```python
from build123d import *

# Parameters (mm, degrees)
SKETCH1_W           = 160
SKETCH1_H           = 100
BOSS_EXTRUDE2_DEPTH = 50
CUT_EXTRUDE2_DEPTH  = 50
CUT_EXTRUDE3_DEPTH  = 50
CUT_EXTRUDE4_DEPTH  = 20
CUT_EXTRUDE5_DEPTH  = 20
SKETCH8_W           = 40
SKETCH8_H           = 10
CUT_EXTRUDE6_DEPTH  = 125
SKETCH9_R           = 35
BOSS_EXTRUDE3_DEPTH = 10
SKETCH10_R          = 15
CUT_EXTRUDE8_DEPTH  = 123
SKETCH11_R          = 35
BOSS_EXTRUDE4_DEPTH = 30
SKETCH12_R          = 15
CUT_EXTRUDE9_DEPTH  = 30
SKETCH13_R          = 20
CUT_EXTRUDE10_DEPTH = 30
CUT_EXTRUDE11_DEPTH = 20
SKETCH15_R          = 20
SKETCH15_R_2        = 15
CUT_EXTRUDE12_DEPTH = 10


with BuildPart() as part:
    # Sketch1 → Boss-Extrude2 (new body)
    with BuildSketch(Plane.XY):
        with Locations((80, 50)):
            Rectangle(SKETCH1_W, SKETCH1_H)
    extrude(amount=BOSS_EXTRUDE2_DEPTH)

    # Sketch4 → Cut-Extrude2 (cut)
    with BuildSketch(Plane.XY.offset(50)):
        Polygon((0, 80), (20, 100), (0, 100), align=None)
        Polygon((0, 20), (20, 0), (0, 0), align=None)
        Polygon((140, 100), (160, 80), (160, 100), align=None)
        Polygon((160, 20), (140, 0), (160, 0), align=None)
    extrude(amount=-CUT_EXTRUDE2_DEPTH, mode=Mode.SUBTRACT)

    # Sketch5 → Cut-Extrude3 (cut)
    with BuildSketch(Plane.XY.offset(50)):
        Polygon((10, 70), (0, 70), (0, 30), (10, 30), (10, 40), (30, 40), (30, 60), (10, 60), align=None)
        Polygon((160, 30), (160, 70), (150, 70), (150, 60), (130, 60), (130, 40), (150, 40), (150, 30), align=None)
    extrude(amount=-CUT_EXTRUDE3_DEPTH, mode=Mode.SUBTRACT)

    # Sketch6 → Cut-Extrude4 (cut)
    with BuildSketch(Plane.XY.offset(50)):
        Polygon((10, 70), (40, 70), (40, 30), (10, 30), (10, 40), (30, 40), (30, 60), (10, 60), align=None)
    extrude(amount=-CUT_EXTRUDE4_DEPTH, mode=Mode.SUBTRACT)

    # Sketch7 → Cut-Extrude5 (cut)
    with BuildSketch(Plane.XY.offset(50)):
        Polygon((150, 70), (120, 70), (120, 30), (150, 30), (150, 40), (130, 40), (130, 60), (150, 60), align=None)
    extrude(amount=-CUT_EXTRUDE5_DEPTH, mode=Mode.SUBTRACT)

    # Sketch8 → Cut-Extrude6 (cut)
    with BuildSketch(Plane.XY.offset(50)):
        with Locations((80, 95)):
            Rectangle(SKETCH8_W, SKETCH8_H)
        with Locations((80, 5)):
            Rectangle(SKETCH8_W, SKETCH8_H)
    extrude(amount=-CUT_EXTRUDE6_DEPTH, mode=Mode.SUBTRACT)

    # Sketch9 → Boss-Extrude3 (add)
    with BuildSketch(Plane(origin=(0, 0, 0), x_dir=(-1, 0, 0), z_dir=(0, 0, -1))):
        with Locations((-80, 50)):
            Circle(SKETCH9_R)
    extrude(amount=BOSS_EXTRUDE3_DEPTH)

    # Sketch10 → Cut-Extrude8 (cut)
    with BuildSketch(Plane(origin=(0, 0, -10), x_dir=(-1, 0, 0), z_dir=(0, 0, -1))):
        with Locations((-80, 50)):
            Circle(SKETCH10_R)
    extrude(amount=-CUT_EXTRUDE8_DEPTH, mode=Mode.SUBTRACT)

    # Sketch11 → Boss-Extrude4 (add)
    with BuildSketch(Plane.XY.offset(50)):
        with Locations((80, 50)):
            Circle(SKETCH11_R)
    extrude(amount=BOSS_EXTRUDE4_DEPTH)

    # Sketch12 → Cut-Extrude9 (cut)
    with BuildSketch(Plane(origin=(0, 0, 50), x_dir=(-1, 0, 0), z_dir=(0, 0, -1))):
        with Locations((-80, 50)):
            Circle(SKETCH12_R)
    extrude(amount=-CUT_EXTRUDE9_DEPTH, mode=Mode.SUBTRACT)

    # Sketch13 → Cut-Extrude10 (cut)
    with BuildSketch(Plane.XY.offset(80)):
        with Locations((80, 50)):
            Circle(SKETCH13_R)
    extrude(amount=-CUT_EXTRUDE10_DEPTH, mode=Mode.SUBTRACT)

    # Sketch14 → Cut-Extrude11 (cut)
    with BuildSketch(Plane.XY.offset(80)):
        with BuildLine():
            ThreePointArc((66.771243445, 35), (60, 50), (66.771243445, 65))
            Line((66.771243445, 65), (48.377223398, 65))
            ThreePointArc((48.377223398, 65), (45, 50), (48.377223398, 35))
            Line((48.377223398, 35), (66.771243445, 35))
        make_face()
        with BuildLine():
            Line((111.622776602, 65), (93.228756555, 65))
            ThreePointArc((93.228756555, 65), (98.228756555, 58.228756555), (100, 50))
            ThreePointArc((100, 50), (98.228756555, 41.771243445), (93.228756555, 35))
            Line((93.228756555, 35), (111.622776602, 35))
            ThreePointArc((111.622776602, 35), (114.145257219, 42.312255892), (115, 50))
            ThreePointArc((115, 50), (114.145257219, 57.687744108), (111.622776602, 65))
        make_face()
    extrude(amount=-CUT_EXTRUDE11_DEPTH, mode=Mode.SUBTRACT)

    # Sketch15 → Cut-Extrude12 (cut)
    with BuildSketch(Plane.XY.offset(50)):
        with Locations((80, 50)):
            Circle(SKETCH15_R)
        with Locations((80, 50)):
            Circle(SKETCH15_R_2, mode=Mode.SUBTRACT)
    extrude(amount=-CUT_EXTRUDE12_DEPTH, mode=Mode.SUBTRACT)


solid = part.part
```
For this review, take the finished solid that the model builds, in its own axes (mm). A direction names the side the tool comes from. Coordinates: 2 decimals unless noted, no trailing zeros. Loops run counter-clockwise (first coordinate to the right, second up) from the corner with the lowest first, then second, coordinate; pieces in that order, holes last.
1. Add section B-B, the plane x = 16.5. Give the boundary of the cut face in (y, z), then the cut area to 3 significant figures.
2. Add section D-D, the plane z = 35.5. Give the boundary of the cut face in (x, y), then the cut area to 3 significant figures.
3. Add section A-A, the plane z = 73.5. Give the boundary of the cut face in (x, y), then the cut area to 3 significant figures.
4. Insertion check: P1, Ø3, axis at y = 4, z = 19, coming from the +X side; P2, Ø3, axis at y = 37, z = 12.5, coming from the +X side; P3, Ø22, axis at x = 21.5, z = 17.5, coming from the -Y side; P4, Ø1.5, axis at y = 69.5, z = 59.5, coming from the +X side. Each pin has a flat end and moves straight along its axis. Give the tip position at first contact, or say it passes through.
5. For faces 1 (the flat face through (128, 50, 30)), 2 (the flat face through (100, 5, 25)), 3 (the flat face through (103, 65, 70)), 4 (the flat face through (30, 50, 15)), 5 (the flat face through (150, 35, 15)), list the 3-axis set-ups (+Z, -Z, +X, -X, +Y, -Y) from which the entire face can be reached by the end or side of a thin tool; tool diameter is ignored.
6. For line 1 (X direction, y = 50, z = 56); line 2 (Y direction, x = 80, z = 61.5); line 3 (Y direction, x = 80, z = 11), list the stretches that pass through material, from the lowest coordinate up.
7. Add section C-C, the plane y = 50. Give the boundary of the cut face in (x, z).
8. Mouldability with a two-part tool opening along Y and no side actions: class faces 6 (the flat face through (145, 70, 36)), 7 (the cylindrical face through (61.18, 79.51, -4.93)), 8 (the flat face through (160, 75, 25)), 9 (the cylindrical face through (71.94, 62.65, 14.65)) as +Y half, -Y half, draft (parallel to the pull), parting line (faces both ways), or undercut.
Result:
1. outline: (3.5, 0) - (40, 0) - (40, 30) - (30, 30) - (30, 50) - (3.5, 50) - close; (60, 0) - (96.5, 0) - (96.5, 50) - (70, 50) - (70, 30) - (60, 30) - close
1. area: 3,250 mm2
2. outline: (0, 20) - (20, 0) - (60, 0) - (60, 10) - (100, 10) - (100, 0) - (140, 0) - (160, 20) - (160, 30) - (120, 30) - (120, 70) - (160, 70) - (160, 80) - (140, 100) - (100, 100) - (100, 90) - (60, 90) - (60, 100) - (20, 100) - (0, 80) - (0, 70) - (40, 70) - (40, 30) - (0, 30) - close; hole circle Ø30 at (80, 50)
2. area: 10,500 mm2
3. outline: (48.38, 35) arc R35 ccw to (111.62, 35) - (93.23, 35) arc R20 cw to (66.77, 35) - close; (48.38, 65) - (66.77, 65) arc R20 cw to (93.23, 65) - (111.62, 65) arc R35 ccw to start
3. area: 1,630 mm2
4. P1: stops at x = 145.5
4. P2: stops at x = 150
4. P3: stops at y = 0
4. P4: stops at x = 109.55
5. face 1: +Z, +X
5. face 2: +Z, -Z, -Y
5. face 3: +Z, +X, -X
5. face 4: +Z, -Z, -X
5. face 5: +Z, -Z, +X
6. line 1: x = 45 to 60, 100 to 115
6. line 2: y = 15 to 30, 70 to 85
6. line 3: y = 10 to 35, 65 to 90
7. outline: (30, 0) - (45, 0) - (45, -10) - (65, -10) - (65, 40) - (60, 40) - (60, 60) - (45, 60) - (45, 50) - (40, 50) - (40, 30) - (30, 30) - close; (95, -10) - (115, -10) - (115, 0) - (130, 0) - (130, 30) - (120, 30) - (120, 50) - (115, 50) - (115, 60) - (100, 60) - (100, 40) - (95, 40) - close
8. face 6: undercut
8. face 7: parting line
8. face 8: draft
8. face 9: undercut
